from build123d import *

# Parameters (mm, degrees)
F0_R     = 2
F0_R_2   = 1
F1_DEPTH = 1.5
F2_DEPTH = 2.5
F3_W     = 5
F3_H     = 2.5
F3_H_2   = 3.5
F4_DEPTH = 1.5
F5_SIZE2 = 2.49999
F5_SIZE  = 1.49999
F6_SIZE2 = 1.49999
F6_SIZE  = 2.49999
F7_DEPTH = 25
F8_DEPTH = 1


# Not quite as in the source:
# - a fillet or chamfer is up to 0.001 mm smaller than in the source, because OpenCascade refuses the exact size
# - a feature names something its author has since deleted; it is built from what else it names


with BuildPart() as f1:
    # F0 (on Top) → F1 (new body)
    with BuildSketch(Plane.XY):
        Polygon((-16.75, 0), (0, 0), (16.75, 0), (16.75, 51.5), (3.6, 51.5), (0, 51.5), (-3.6, 51.5), (-16.75, 51.5), align=None)
        with BuildLine():
            ThreePointArc((3.6, 55.4), (0, 59), (-3.6, 55.4))
            ThreePointArc((-3.6, 55.4), (0, 51.8), (3.6, 55.4))
        make_face()
        with Locations((0, 55.4)):
            Circle(F0_R, mode=Mode.SUBTRACT)
        with Locations((0, 55.4)):
            Circle(F0_R)
        with Locations((0, 55.4)):
            Circle(F0_R_2, mode=Mode.SUBTRACT)
        with BuildLine():
            Line((-3.6, 55.4), (-3.6, 51.5))
            Line((-3.6, 51.5), (0, 51.5))
            Line((0, 51.5), (3.6, 51.5))
            Line((3.6, 51.5), (3.6, 55.4))
            ThreePointArc((3.6, 55.4), (0, 51.8), (-3.6, 55.4))
        make_face()
        with Locations((0, 55.4)):
            Circle(F0_R_2)
    extrude(amount=F1_DEPTH)

    # F0 (on Top) → F2 (join)
    with BuildSketch(Plane.XY):
        with BuildLine():
            ThreePointArc((3.6, 55.4), (0, 59), (-3.6, 55.4))
            ThreePointArc((-3.6, 55.4), (0, 51.8), (3.6, 55.4))
        make_face()
        with Locations((0, 55.4)):
            Circle(F0_R, mode=Mode.SUBTRACT)
        with Locations((0, 55.4)):
            Circle(F0_R)
        with Locations((0, 55.4)):
            Circle(F0_R_2, mode=Mode.SUBTRACT)
        with Locations((0, 55.4)):
            Circle(F0_R_2)
    extrude(amount=F2_DEPTH)

    # F3 (on face) → F4 (join)
    with BuildSketch(Plane.XY.offset(1.5)):
        with Locations((-10.2441851608, -1.25)):
            Rectangle(F3_W, F3_H)
        with Locations((-10.2441851608, 1.75)):
            Rectangle(F3_W, F3_H_2)
        with Locations((10.2441851608, -1.25)):
            Rectangle(F3_W, F3_H)
        with Locations((10.2441851608, 1.75)):
            Rectangle(F3_W, F3_H_2)
    extrude(amount=F4_DEPTH)

    # F5 (size 1.5 and 2.5 in the source; OpenCascade refuses exactly that, so slightly less here)
    f5_edges = [f1.edges().sort_by_distance(p)[0] for p in [
        (-10.244185, -2.5, 3),
    ]]
    f5_side = f1.faces().sort_by_distance((-10.244185, -2.5, 2.25))[0]
    chamfer(f5_edges, length=F5_SIZE, length2=F5_SIZE2, reference=f5_side)

    # F6 (size 2.5 and 1.5 in the source; OpenCascade refuses exactly that, so slightly less here)
    f6_edges = [f1.edges().sort_by_distance(p)[0] for p in [
        (10.244185, -2.5, 3),
    ]]
    f6_side = f1.faces().sort_by_distance((10.244185, 0.5, 3))[0]
    chamfer(f6_edges, length=F6_SIZE, length2=F6_SIZE2, reference=f6_side)

    # F0 (on Top) → F7 (cut)
    with BuildSketch(Plane.XY):
        with Locations((0, 55.4)):
            Circle(F0_R_2)
    extrude(amount=F7_DEPTH, mode=Mode.SUBTRACT)

    # F0 (on Top) → F8 (cut)
    with BuildSketch(Plane.XY):
        with Locations((0, 55.4)):
            Circle(F0_R)
        with Locations((0, 55.4)):
            Circle(F0_R_2, mode=Mode.SUBTRACT)
    extrude(amount=F8_DEPTH, mode=Mode.SUBTRACT)


solid = f1.part
The model under review builds one solid part; all positions refer to its coordinate system, in mm. A direction names the side the tool comes from. Round coordinates to 2 decimals unless told otherwise and drop trailing zeros. Order: outer loops, then holes, each group sorted by start corner. A loop starts at its lowest first (then second) coordinate and runs counter-clockwise, first axis right, second up. Notation, with made-up numbers: (69.5, 1.5) -> (94.5, 1.5) arc R21 ccw to (94.5, 19.5) -> close; hole circle Ø7 at (-10, 81). An arc over 180 degrees is marked (long way). Use CSV: the item, a comma, the result in double quotes. Start each with the question number.
(1) Consider section A-A on x = 0. Write out the cut boundary in (y, z).
(2) Mouldability with a two-part tool opening along Y and no side actions: class faces 1 (the face through (-10, 51.5, 1)), 2 (the face through (10, -1, 1.5)), 3 (the face through (0.923, 53.626, 0.493)) as pulls with the +Y half, pulls with the -Y half, needs draft (parallel to the pull), parting line crosses it, or undercut.
(3) Tool access review of faces 4 (the face through (3.6, 53, 1)), 5 (the face through (-1, 56, 1)), 6 (the face through (10, 3.5, 2)): name each direction out of +Z, -Z, +X, -X, +Y, -Y from which nothing blocks a thin tool from reaching the whole face with its end or side.
(4) Consider section D-D on x = 6. Write out the cut boundary in (y, z).
(5) Consider section C-C on y = 24. Write out the cut boundary in (x, z).
(6) Insertion check: pin 1 (0.8 mm diameter, centred on x = 7, z = 1, fed in from -Y); pin 2 (1.6 mm diameter, centred on x = -9.5, z = 1, fed in from +Y); pin 3 (1.2 mm diameter, centred on y = 0.5, z = 2.5, fed in from -X). Each pin has a flat end and moves straight along its axis. Give the tip position at first contact, or say it passes through.
(7) Wall thickness on probe 1 along Z at (x, y) = (14, 4); probe 2 along Y at (x, z) = (-7, 0.5); probe 3 along Y at (x, z) = (-2.5, 0.35): over which ranges is each line inside the solid? List them lowest first. Write a range as from..to.
Responses:
1,outline,"(0, 0) -> (53.4, 0) -> (53.4, 1) -> (54.4, 1) -> (54.4, 2.5) -> (51.8, 2.5) -> (51.8, 1.5) -> (0, 1.5) -> close; (56.4, 1) -> (57.4, 1) -> (57.4, 0) -> (59, 0) -> (59, 2.5) -> (56.4, 2.5) -> close"
2,face 1,"pulls with the +Y half"
2,face 2,"needs draft"
2,face 3,"undercut"
3,face 4,"+Z, -Z, +X, +Y"
3,face 5,"-Z"
3,face 6,"+Z, +X, -X, +Y"
4,outline,"(0, 0) -> (51.5, 0) -> (51.5, 1.5) -> (0, 1.5) -> close"
5,outline,"(-16.75, 0) -> (16.75, 0) -> (16.75, 1.5) -> (-16.75, 1.5) -> close"
6,pin 1,"y = 0"
6,pin 2,"y = 51.5"
6,pin 3,"x = -12.74"
7,probe 1,"0..1.5"
7,probe 2,"0..51.5"
7,probe 3,"0..57.99"
